Build history of the part. All positions in model axes, mm. Face numbers are marked on the shaded views. A direction names the side the tool comes from. Give positions to 0.01 mm unless a question says otherwise; leave off trailing zeros. Loops run counter-clockwise (first coordinate to the right, second up) from the corner with the lowest first, then second, coordinate; pieces in that order, holes last. Notation, with made-up numbers: (-12.5, 21) -> (-3.5, 21) arc R33 cw to (-3.5, 59) -> close; hole circle Ø7 at (8, 87.5). An arc over 180 degrees is marked (long way). One line per question, with ' | ' between items. Start each with the question number.
(1) Slice it at C-C, the plane y = 17.5. Write the cut outline in (x, z), then the cut area to 3 significant figures.
(2) 3-axis set-ups, long thin cutter, end or side, ignore diameter. For the marked faces 1, 2, 3 and 4: which of +Z, -Z, +X, -X, +Y, -Y reach the whole face in a straight line?
(3) Drill centre lines: L1, parallel to X at y = 6.5, z = 5; L2, parallel to Y at x = -2.5, z = 7.9; L3, parallel to Z at x = 11.25, y = 11.5. Where is each one in solid material? Low to high. Write a range as from..to.
(4) Slice it at A-A, the plane z = 6.5. Write the cut outline in (x, y).
(5) Slice it at B-B, the plane z = 25. Write the cut outline in (x, y).
(6) Slice it at D-D, the plane x = 6. Write the cut outline in (y, z), then the cut area to 3 significant figures.
(7) Mould opens along X. For the marked faces 5, 6, 7 and 8 say: pulls with the +X half, pulls with the -X half, needs draft (parallel to the pull), parting line crosses it, or undercut.
(8) Flat gauge pins, fed straight in: pin 1 Ø4 at (x, y) = (6.5, 7) entering from -Z; pin 2 Ø4.5 at (x, y) = (14.74, 17.5) entering from -Z; pin 3 Ø2 at (x, z) = (5, 27.5) entering from -Y. Where does each tip first touch, or does it go through?
```python
from build123d import *

# Parameters (mm, degrees)
CYLINDER004_R     = 2.4
CYLINDER004_DEPTH = 13
CYLINDER005_R     = 2.7
CYLINDER005_DEPTH = 1
CYLINDER006_R     = 2.7
CYLINDER006_DEPTH = 1
CYLINDER003_R     = 2.4
CYLINDER003_DEPTH = 13
CYLINDER002_R     = 0.7
CYLINDER002_DEPTH = 16
BOX007_W          = 12.25
BOX007_H          = 10
BOX007_DEPTH      = 10
BOX003_W          = 12.25
BOX003_H          = 23.78
BOX003_DEPTH      = 22.68
BOX008_W          = 24.3
BOX008_H          = 21
BOX008_DEPTH      = 30


with BuildPart() as cylinder004:
    # Cylinder004 → Cylinder004 (new body)
    with BuildSketch(Plane(origin=(14.74, 17.5, -6.5), x_dir=(1, 0, 0), z_dir=(0, 0, 1))):
        Circle(CYLINDER004_R)
    extrude(amount=CYLINDER004_DEPTH)


with BuildPart() as cylinder005:
    # Cylinder005 → Cylinder005 (new body)
    with BuildSketch(Plane(origin=(-2.5, 17.5, 6.5), x_dir=(1, 0, 0), z_dir=(0, 0, 1))):
        Circle(CYLINDER005_R)
    extrude(amount=CYLINDER005_DEPTH)


with BuildPart() as cylinder006:
    # Cylinder006 → Cylinder006 (new body)
    with BuildSketch(Plane(origin=(14.74, 17.5, 6.5), x_dir=(1, 0, 0), z_dir=(0, 0, 1))):
        Circle(CYLINDER006_R)
    extrude(amount=CYLINDER006_DEPTH)


with BuildPart() as fusion004:
    # Cylinder003 → Cylinder003 (new body)
    with BuildSketch(Plane(origin=(-2.5, 17.5, -6.5), x_dir=(1, 0, 0), z_dir=(0, 0, 1))):
        Circle(CYLINDER003_R)
    extrude(amount=CYLINDER003_DEPTH)

    # Fusion004: union Cylinder004, Cylinder005, Cylinder006
    add(cylinder004.part)
    add(cylinder005.part)
    add(cylinder006.part)


with BuildPart() as fusion004_1:
    # Fusion004 placement: moved
    add(fusion004.part.moved(Location((0, 0, 1))))


with BuildPart() as cylinder002:
    # Cylinder002 → Cylinder002 (new body)
    with BuildSketch(Plane(origin=(6, 22, 25), x_dir=(1, 0, 0), z_dir=(0, -1, 0))):
        Circle(CYLINDER002_R)
    extrude(amount=CYLINDER002_DEPTH)


with BuildPart() as cube004:
    # Box007 → Box007 (new body)
    with BuildSketch(Plane(origin=(0, -3.25, 22), x_dir=(1, 0, 0), z_dir=(0, 0, 1))):
        with Locations((6.125, 5)):
            Rectangle(BOX007_W, BOX007_H)
    extrude(amount=BOX007_DEPTH)


with BuildPart() as servo002:
    # Box003 → Box003 (new body)
    with BuildSketch(Plane(origin=(0, -1, 0), x_dir=(1, 0, 0), z_dir=(0, 0, 1))):
        with Locations((6.125, 11.89)):
            Rectangle(BOX003_W, BOX003_H)
    extrude(amount=BOX003_DEPTH)

    # Fusion002: union Cube004
    add(cube004.part)


with BuildPart() as fusion003:
    # Fusion003 base: copy of Cube004
    add(cube004.part)

    # Fusion003: union servo002
    add(servo002.part)


with BuildPart() as cut004:
    # Box008 → Box008 (new body)
    with BuildSketch(Plane(origin=(-6, 0, 0), x_dir=(1, 0, 0), z_dir=(0, 0, 1))):
        with Locations((12.15, 10.5)):
            Rectangle(BOX008_W, BOX008_H)
    extrude(amount=BOX008_DEPTH)

    # Cut002: cut Fusion003
    add(fusion003.part, mode=Mode.SUBTRACT)

    # Cut003: cut Cylinder002
    add(cylinder002.part, mode=Mode.SUBTRACT)

    # Cut004: cut Fusion004
    add(fusion004_1.part, mode=Mode.SUBTRACT)


solid = cut004.part
```
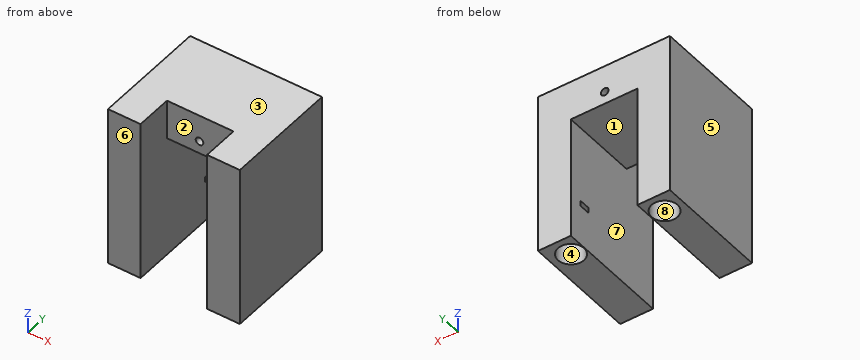
Final values:
1) outline: (-6, 0) -> (-4.9, 0) -> (-4.9, 7.5) -> (-5.2, 7.5) -> (-5.2, 8.5) -> (0, 8.5) -> (0, 22.68) -> (12.25, 22.68) -> (12.25, 8.5) -> (17.44, 8.5) -> (17.44, 7.5) -> (17.14, 7.5) -> (17.14, 0) -> (18.3, 0) -> (18.3, 30) -> (-6, 30) -> close; (-0.1, 0) -> (0, 0) -> (0, 7.5) -> (-0.1, 7.5) -> close; (12.25, 0) -> (12.34, 0) -> (12.34, 7.5) -> (12.25, 7.5) -> close; hole circle Ø1.4 at (6, 25) | area: 367 mm2
2) face 1: -Z, +Y, -Y | face 2: +Z, -Z, -Y | face 3: +Z, +X, -X, +Y, -Y | face 4: -Z
3) L1: -6..0, 12.25..18.3 | L2: 0..14.8, 20.2..21 | L3: 22.68..30
4) outline: (-6, 0) -> (0, 0) -> (0, 21) -> (-6, 21) -> close; (12.25, 0) -> (18.3, 0) -> (18.3, 21) -> (12.25, 21) -> close; hole circle Ø4.8 at (-2.5, 17.5); hole circle Ø4.8 at (14.74, 17.5)
5) outline: (-6, 0) -> (0, 0) -> (0, 6.75) -> (5.3, 6.75) -> (5.3, 21) -> (-6, 21) -> close; (6.7, 6.75) -> (12.25, 6.75) -> (12.25, 0) -> (18.3, 0) -> (18.3, 21) -> (6.7, 21) -> close
6) outline: (6.75, 22.68) -> (21, 22.68) -> (21, 24.3) -> (6.75, 24.3) -> close; (6.75, 25.7) -> (21, 25.7) -> (21, 30) -> (6.75, 30) -> close | area: 84.4 mm2
7) face 5: pulls with the -X half | face 6: needs draft | face 7: undercut | face 8: undercut
8) pin 1: z = 22.68 | pin 2: z = 8.5 | pin 3: y = 6.75
